from build123d import *

# Parameters (mm, degrees)
SKETCH1_W           = 19.05
SKETCH1_H           = 44.45
BOSS_EXTRUDE1_DEPTH = 9.525
SKETCH2_R           = 2.0193
CUT_EXTRUDE1_DEPTH  = 9.525
SKETCH3_R           = 2.0193
CUT_EXTRUDE2_DEPTH  = 9.525
SKETCH4_R           = 2.0193
CUT_EXTRUDE3_DEPTH  = 6.35
SKETCH5_R           = 2.0193
CUT_EXTRUDE4_DEPTH  = 6.35
SKETCH6_R           = 2.0193
CUT_EXTRUDE5_DEPTH  = 6.35
FILLET1_R           = 2.54


with BuildPart() as part:
    # Sketch1 → Boss-Extrude1 (new body, symmetric)
    with BuildSketch(Plane(origin=(0, 0, 0), x_dir=(1, 0, 0), z_dir=(0, 1, 0))):
        Rectangle(SKETCH1_W, SKETCH1_H)
    extrude(amount=BOSS_EXTRUDE1_DEPTH, both=True)

    # Sketch2 → Cut-Extrude1 (cut)
    with BuildSketch(Plane.XY.offset(22.225)):
        Circle(SKETCH2_R)
    extrude(amount=-CUT_EXTRUDE1_DEPTH, mode=Mode.SUBTRACT)

    # Sketch3 → Cut-Extrude2 (cut)
    with BuildSketch(Plane(origin=(0, 0, -22.225), x_dir=(-1, 0, 0), z_dir=(0, 0, -1))):
        Circle(SKETCH3_R)
    extrude(amount=-CUT_EXTRUDE2_DEPTH, mode=Mode.SUBTRACT)

    # Sketch4 → Cut-Extrude3 (cut)
    with BuildSketch(Plane(origin=(9.525, 0, 0), x_dir=(0, 0, -1), z_dir=(1, 0, 0))):
        with Locations((-12.7, 3.175)):
            Circle(SKETCH4_R)
        with Locations((12.7, 3.175)):
            Circle(SKETCH4_R)
        with Locations((0, 3.175)):
            Circle(SKETCH4_R)
    extrude(amount=-CUT_EXTRUDE3_DEPTH, mode=Mode.SUBTRACT)

    # Sketch5 → Cut-Extrude4 (cut)
    with BuildSketch(Plane.ZY.offset(9.525)):
        with Locations((-12.7, 3.175)):
            Circle(SKETCH5_R)
        with Locations((0, 3.175)):
            Circle(SKETCH5_R)
        with Locations((12.7, 3.175)):
            Circle(SKETCH5_R)
    extrude(amount=-CUT_EXTRUDE4_DEPTH, mode=Mode.SUBTRACT)

    # Sketch6 → Cut-Extrude5 (cut)
    with BuildSketch(Plane(origin=(0, 9.525, 0), x_dir=(1, 0, 0), z_dir=(0, 1, 0))):
        with Locations((0, 12.7)):
            Circle(SKETCH6_R)
        Circle(SKETCH6_R)
        with Locations((0, -12.7)):
            Circle(SKETCH6_R)
    extrude(amount=-CUT_EXTRUDE5_DEPTH, mode=Mode.SUBTRACT)

    # Fillet1
    fillet1_edges = [part.edges().sort_by_distance(p)[0] for p in [
        (9.525, 0, 22.225),
        (-9.525, 0, 22.225),
        (-9.525, 0, -22.225),
        (9.525, 0, -22.225),
    ]]
    fillet(fillet1_edges, radius=FILLET1_R)


solid = part.part
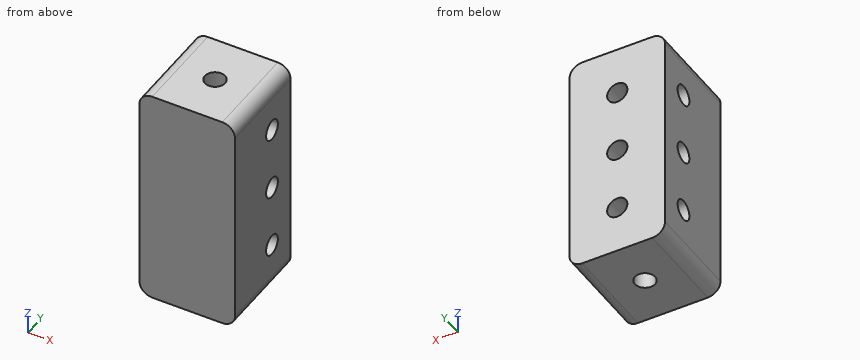
The listing builds one solid part. Answer for the finished solid, in the listing's coordinates (mm). Coordinates: 2 decimals unless noted, no trailing zeros. Order: outer loops, then holes, each group sorted by start corner. A loop starts at its lowest first (then second) coordinate and runs counter-clockwise, first axis right, second up. Notation, with made-up numbers: (40, 75.5) -> (79, 75.5) arc R36 ccw to (79, 114.5) -> close; hole circle Ø1 at (32, 61). An arc over 180 degrees is marked (long way). Answer in a Markdown table with one row per item. Add a question column.
Item 1: Find section B-B (z = 0). Write down the section's boundary in (x, y) (3 decimals), then the cut area to 3 significant figures.
Item 2: Find section C-C (x = 5.75). Write down the section's boundary in (y, z) (3 decimals), then the cut area to 3 significant figures.
Item 3: Find the intervals of material crossed by L1, parallel to Z at x = 0, y = 5.75 (3 decimals); L2, parallel to Y at x = 7.5, z = -12.7 (3 decimals), in increasing order. Write a range as from..to.
Item 4: Find section A-A (x = 0). Write down the section's boundary in (y, z) (3 decimals).
Item 5: Find section D-D (y = 0). Write down the section's boundary in (x, z) (3 decimals), then the cut area to 3 significant figures.
Item 6: Each of these flat-tipped pins is pushed along its axis until it touches: P1, Ø3, axis at y = 3.175, z = -12.7, coming from the +X side (3 decimals); P2, Ø2, axis at x = -0.5, z = 12.5, coming from the +Y side (3 decimals); P3, Ø3.5, axis at x = 0, y = 0, coming from the +Z side. Where does it stop, or does it pass through?
Result set:
| question | item | result |
|---|---|---|
| 1 | outline | (-9.525, -9.525) -> (9.525, -9.525) -> (9.525, 1.156) -> (3.175, 1.156) -> (3.175, 5.194) -> (9.525, 5.194) -> (9.525, 9.525) -> (2.019, 9.525) -> (2.019, 3.175) -> (-2.019, 3.175) -> (-2.019, 9.525) -> (-9.525, 9.525) -> (-9.525, 5.194) -> (-3.175, 5.194) -> (-3.175, 1.156) -> (-9.525, 1.156) -> close |
| 1 | area | 286 mm² |
| 2 | outline | (-9.525, -22.225) -> (9.525, -22.225) -> (9.525, 22.225) -> (-9.525, 22.225) -> close; hole circle Ø4.039 at (3.175, -12.7); hole circle Ø4.039 at (3.175, 0); hole circle Ø4.039 at (3.175, 12.7) |
| 2 | area | 808 mm² |
| 3 | L1 | z = -22.225..-14.719, -10.681..-2.019, 2.019..10.681, 14.719..22.225 |
| 3 | L2 | y = -9.525..1.156, 5.194..9.525 |
| 4 | outline | (-9.525, -22.225) -> (-2.019, -22.225) -> (-2.019, -12.7) -> (2.019, -12.7) -> (2.019, -22.225) -> (9.525, -22.225) -> (9.525, -14.719) -> (3.175, -14.719) -> (3.175, -10.681) -> (9.525, -10.681) -> (9.525, -2.019) -> (3.175, -2.019) -> (3.175, 2.019) -> (9.525, 2.019) -> (9.525, 10.681) -> (3.175, 10.681) -> (3.175, 14.719) -> (9.525, 14.719) -> (9.525, 22.225) -> (2.019, 22.225) -> (2.019, 12.7) -> (-2.019, 12.7) -> (-2.019, 22.225) -> (-9.525, 22.225) -> close |
| 5 | outline | (-9.525, -19.685) arc R2.54 ccw to (-6.985, -22.225) -> (-2.019, -22.225) -> (-2.019, -12.7) -> (2.019, -12.7) -> (2.019, -22.225) -> (6.985, -22.225) arc R2.54 ccw to (9.525, -19.685) -> (9.525, 19.685) arc R2.54 ccw to (6.985, 22.225) -> (2.019, 22.225) -> (2.019, 12.7) -> (-2.019, 12.7) -> (-2.019, 22.225) -> (-6.985, 22.225) arc R2.54 ccw to (-9.525, 19.685) -> close |
| 5 | area | 764 mm² |
| 6 | P1 | stops at x = 3.175 |
| 6 | P2 | stops at y = 3.175 |
| 6 | P3 | stops at z = 12.7 |
